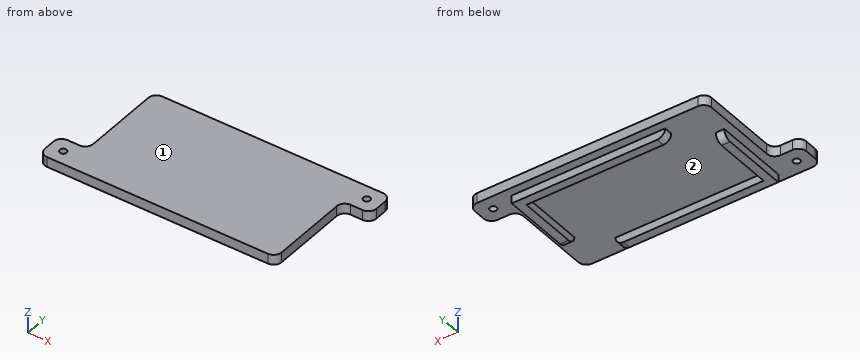
Autodesk Inventor part; units mm, degrees
ref_plane "YZ Plane" through (0, 0, 0) normal (1, 0, 0) x (0, 1, 0)
ref_plane "XZ Plane" through (0, 0, 0) normal (0, 1, 0) x (-1, 0, 0)
ref_plane "XY Plane" through (0, 0, 0) normal (0, 0, 1) x (1, 0, 0)
sketch "Эскиз1" plane through (0, 0, 0) normal (0, 0, 1) x (1, 0, 0)
  line L0 (-21.8917, 12.7106) -> (30.1083, 12.7106)
  line L1 (30.1083, 5.7106) -> (30.1083, -17.2894)
  line L2 (30.1083, -17.2894) -> (-21.8917, -17.2894)
  line L3 (-21.8917, -10.2894) -> (-21.8917, 12.7106)
  line L4 (-21.8917, -17.2894) -> (-28.8917, -17.2894)
  line L5 (-28.8917, -17.2894) -> (-28.8917, -10.2894)
  line L6 (-28.8917, -10.2894) -> (-21.8917, -10.2894)
  line L7 (30.1083, 12.7106) -> (37.1083, 12.7106)
  line L8 (37.1083, 12.7106) -> (37.1083, 5.7106)
  line L9 (37.1083, 5.7106) -> (30.1083, 5.7106)
  point P0 (0, 0)
  dimension "d3" = 7
  dimension "d5" = 7
extrude "Выдавливание1" add sketch "Эскиз1" along normal blind 2.5
fillet "Сопряжение1" radius 2 6 edges at (37.1083, 12.7106, 1.25) (37.1083, 5.7106, 1.25) (30.1083, -17.2894, 1.25) (-28.8917, -10.2894, 1.25) (-21.8917, 12.7106, 1.25) (-28.8917, -17.2894, 1.25)
fillet "Сопряжение2" radius 2 2 edges at (-21.8917, -10.2894, 1.25) (30.1083, 5.7106, 1.25)
sketch "Эскиз2" plane through (0, 0, 2.5) normal (0, 0, 1) x (1, 0, 0)
  arc A0 (-26.8917, -10.2894) -> (-28.8917, -12.2894) centre (-26.8917, -12.2894) ccw
  circle A1 centre (-25.3917, -13.7894) radius 0.85
  circle A2 centre (33.6083, 9.2106) radius 0.85
  point P0 (0, 0)
  point P1 (37.1083, 10.7106)
  point P2 (35.1083, 5.7106)
  dimension "d12" = 1.7
  dimension "d15" = 1.7
extrude "Выдавливание2" cut sketch "Эскиз2" against normal blind 2.5
sketch "Эскиз3" plane through (0, 0, 0) normal (0, 0, -1) x (-1, 0, 0)
  arc A0 (21.8917, 10.7106) -> (19.8917, 12.7106) centre (19.8917, 10.7106) ccw
  line L0 (-28.1083, -17.2894) -> (26.8917, -17.2894)
  line L1 (-19.2442, -15.1834) -> (19.7856, -15.1834)
  line L2 (19.7856, -15.1834) -> (19.7856, 3.4434)
  line L3 (10.2125, 10.6045) -> (-28.0023, 10.6045)
  line L4 (-28.0023, 10.6045) -> (-28.0023, -8.0395)
  line L5 (19.7856, -15.1834) -> (22.7856, -15.1834) construction
  line L6 (17.6643, -13.062) -> (-19.2442, -13.062)
  line L7 (-25.8809, -8.0395) -> (-25.8809, 8.4832)
  line L8 (-25.8809, 8.4832) -> (10.2125, 8.4832)
  line L9 (17.6643, 3.4434) -> (17.6643, -13.062)
  line L10 (10.2125, 10.6045) -> (10.2125, 8.4832)
  line L11 (19.7856, 3.4434) -> (17.6643, 3.4434)
  line L12 (-19.2442, -15.1834) -> (-19.2442, -13.062)
  line L13 (-28.0023, -8.0395) -> (-25.8809, -8.0395)
  point P0 (0, 0)
extrude "Выдавливание3" add sketch "Эскиз3" along normal blind 2
fillet "Сопряжение3" radius 2 4 edges at (-18.7249, 3.4434, -2) (-10.2125, 9.5438, -2) (26.9416, -8.0395, -2) (19.2442, -14.1227, -2)
properties part number "Дно Модуля БП"
Model file for the job. Use its own axes, mm. Face numbers are marked on the shaded views. Round coordinates to 2 decimals unless told otherwise and drop trailing zeros. Loops run counter-clockwise (first coordinate to the right, second up) from the corner with the lowest first, then second, coordinate; pieces in that order, holes last. Notation, with made-up numbers: (-5.75, 70) - (48.25, 70) arc R17 ccw to (48.25, 75) - close; hole circle Ø4 at (42.25, 50). An arc over 180 degrees is marked (long way). Write each question's results on one line, items separated by ' | '.
(1) Pin check, flat tips, straight feed: pin 1 (0.6 mm diameter, centred on y = -2, z = -1.5, fed in from +X); pin 2 (2 mm diameter, centred on x = 19.5, y = -9.5, fed in from -Z); pin 3 (1 mm diameter, centred on x = 9, z = -1, fed in from -Y). Stop position of each tip, or through.
Answer below:
pin 1: stops at x = 28 | pin 2: stops at z = 0 | pin 3: stops at y = -15.18
(2) Wall check: L1, parallel to X at y = -1, z = -0.7; L2, parallel to X at y = 0.25, z = 2.15; L3, parallel to Z at x = 24, y = -5. Give the ranges that are in metal, low to high.
Answer below:
L1: x = -19.79 to -17.66, 25.88 to 28 | L2: x = -21.89 to 30.11 | L3: z = 0 to 2.5
(3) Saw through at C-C, the plane y = -7. List the corners of the cut face in (x, z).
Answer below:
outline: (-21.89, 0) - (-19.79, 0) - (-19.79, -2) - (-17.66, -2) - (-17.66, 0) - (25.88, 0) - (25.88, -1.75) - (28, -1.75) - (28, 0) - (30.11, 0) - (30.11, 2.5) - (-21.89, 2.5) - close
(4) Saw through at B-B, the plane x = -1.5. List the corners of the cut face in (y, z), then the cut area to 3 significant figures.
Answer below:
outline: (-17.29, 0) - (-15.18, 0) - (-15.18, -2) - (-13.06, -2) - (-13.06, 0) - (8.48, 0) - (8.48, -2) - (10.6, -2) - (10.6, 0) - (12.71, 0) - (12.71, 2.5) - (-17.29, 2.5) - close | area: 83.5 mm^2
(5) Mould opens along Y. For the marked faces 1 and 2 say: released by +Y, released by -Y, zero draft, split by the parting line, or undercut.
Answer below:
face 1: zero draft | face 2: undercut
(6) Saw through at A-A, the plane z = -0.95. List the corners of the cut face in (x, y).
Answer below:
outline: (-19.79, -15.18) - (19, -15.18) - (19, -13.06) - (-17.66, -13.06) - (-17.66, 3.2) - (-19.79, 3.2) - close; (-9.97, 8.48) - (25.88, 8.48) - (25.88, -7.8) - (28, -7.8) - (28, 10.6) - (-9.97, 10.6) - close
(7) Saw through at D-D, the plane y = 7. List the corners of the cut face in (x, z), then the cut area to 3 significant figures.
Answer below:
outline: (-21.89, 0) - (25.88, 0) - (25.88, -2) - (28, -2) - (28, 0) - (36.98, 0) - (36.98, 2.5) - (-21.89, 2.5) - close | area: 151 mm^2
